For this review, take the finished solid that the model builds, in its own axes (mm). Face numbers are marked on the shaded views. A direction names the side the tool comes from. Give positions to 0.01 mm unless a question says otherwise; leave off trailing zeros. Write each loop counter-clockwise with the first axis right and the second up, starting at its lowest first coordinate (ties: lowest second). Pieces come first, ordered by that corner, then holes.
1) We need section A-A on z = -1. Give the boundary of the cut face in (x, y).
2) We need section B-B on y = -1.5. Give the boundary of the cut face in (x, z).
3) Draft analysis for pull direction Y (two halves, no side actions). For the marked faces 1, 2 and 3, state which applies: pulls with the +Y half, pulls with the -Y half, needs draft (parallel to the pull), parting line crosses it, or undercut.
4) We need section D-D on y = 3.5. Give the boundary of the cut face in (x, z).
5) Machinability: for the marked faces 4 and 5, which of the approach directions +Z, -Z, +X, -X, +Y, -Y give a long, thin tool a straight path to every point of the face, cutting with its end or side? Answer none if there is none.
6) Wall thickness on line 1 along Y through (x, z) = (-19.5, -6); line 2 along X through (y, z) = (0, -1.5); line 3 along Z through (x, y) = (-3, -1.25): over which ranges is each line inside the solid? List them lowest first.
7) For P1, Ø2.5, axis at x = 19.5, y = 0, coming from the -Z side; P2, Ø3.5, axis at y = -2, z = -2, coming from the +X side; P3, Ø1.5, axis at y = -3, z = -1.5, coming from the -X side; P4, Ø2, axis at x = -8.5, y = -3, coming from the +Z side, all flat-tipped, find the tip position at first contact; note any pin that passes through.
8) We need section C-C on x = -11.5. Give the boundary of the cut face in (y, z), and give its area (3 significant figures).
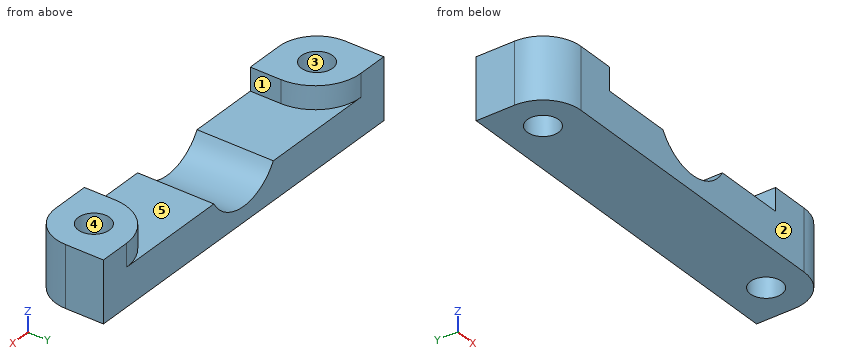
Solid Edge part; units mm, degrees
sketch "Sketch1" plane through (0, 0, 0) normal (0, -1, 0) x (1, 0, 0)
  line L0 (-24.5, 0) -> (-24.5, -8)
  line L1 (-24.5, -8) -> (24.5, -8)
  line L2 (24.5, -8) -> (24.5, 0)
  line L3 (24.5, 0) -> (14.5, 0)
  line L4 (14.5, 0) -> (14.5, -3)
  line L5 (14.5, -3) -> (-14.5, -3)
  line L6 (-14.5, -3) -> (-14.5, 0)
  line L7 (-14.5, 0) -> (-24.5, 0)
  dimension "D1" = 14.5
  dimension "D2" = 24.5
  dimension "D3" = 14.5
  dimension "D4" = 14.5
  dimension "D5" = 14.5
  dimension "D6" = 24.5
  dimension "D7" = 14.5
extrude "Ajout_matière_1" add sketch "Sketch1" along normal mid plane 10
sketch "Sketch2" plane through (0, 0, 0) normal (0, -1, 0) x (1, 0, 0)
  circle A0 centre (0, 0) radius 6
extrude "Cutout1" cut sketch "Sketch2" along normal mid plane 10
hole "Perçage_1" at (-19.5, 0, 0) direction (0, 0, -1) diameter 4.1 end up to next
mirror "Mirror1" about plane through (0, 0, 0) normal (1, 0, 0) of "Perçage_1"
fillet "Congé_1" radius 6 2 edges at (-14.5, 5, -1.5) (14.5, 5, -1.5)
fillet "Congé_2" radius 5 2 edges at (-24.5, -5, -4) (24.5, -5, -4)
properties material "Plastique ABS, performance moyenne"
Results list:
1. outline: (-24.5, 0) arc R5 ccw to (-19.5, -5) - (-14.5, -5) - (-14.5, -1) arc R6 ccw to (-20.5, 5) - (-24.5, 5) - close; (14.5, -5) - (19.5, -5) arc R5 ccw to (24.5, 0) - (24.5, 5) - (20.5, 5) arc R6 ccw to (14.5, -1) - close; hole circle Ø4.1 at (-19.5, 0); hole circle Ø4.1 at (19.5, 0)
2. outline: (-24.27, -8) - (-20.9, -8) - (-20.9, 0) - (-24.27, 0) - close; (-18.1, -8) - (18.1, -8) - (18.1, 0) - (14.5, 0) - (14.5, -3) - (5.2, -3) arc R6 cw to (-5.2, -3) - (-14.5, -3) - (-14.5, 0) - (-18.1, 0) - close; (20.9, -8) - (24.27, -8) - (24.27, 0) - (20.9, 0) - close
3. face 1: needs draft
3. face 2: pulls with the -Y half
3. face 3: undercut
4. outline: (-24.5, -8) - (24.5, -8) - (24.5, 0) - (16.53, 0) - (16.53, -3) - (5.2, -3) arc R6 cw to (-5.2, -3) - (-16.53, -3) - (-16.53, 0) - (-24.5, 0) - close
5. face 4: +Z, -Z
5. face 5: +Z, +Y
6. line 1: y = -5 to -2.05, 2.05 to 5
6. line 2: x = -24.5 to -21.55, -17.45 to -14.58, 14.58 to 17.45, 21.55 to 24.5
6. line 3: z = -8 to -5.2
7. P1: passes through
7. P2: stops at x = 24.49
7. P3: stops at x = -23.97
7. P4: stops at z = -3
8. outline: (-5, -8) - (5, -8) - (5, -3) - (-5, -3) - close
8. area: 50.0 mm2
